Here's how the part is built. I have some questions about the finished solid (model axes, mm). A direction names the side the tool comes from. Round coordinates to 2 decimals unless told otherwise and drop trailing zeros. Write each loop counter-clockwise with the first axis right and the second up, starting at its lowest first coordinate (ties: lowest second). Pieces come first, ordered by that corner, then holes. Notation, with made-up numbers: M 69,18.5 L 109,18.5 A19 ccw 109,44.5 Z; hole C 79.5,49.5 d4. An arc over 180 degrees is marked long. Use one line per item in the form item = value. Start each with the question number.
Q1. I want a section at D-D on x = 25. List the corners of the cut face in (y, z) for me, and give its area (3 significant figures).
Q2. I'm going to push a flat-ended pin straight in: pin 1 Ø1 at (y, z) = (-6.5, -0.5) entering from -X. Where does the tip first touch, or does it pass through?
Q3. I want a section at B-B on y = 0. List the corners of the cut face in (x, z) for me.
Q4. We'd pull the mould along X, two halves only. Please class faces 1 (the face through (-30.745, -1.854, 0.018)), 2 (the face through (26.52, 10.27, 0.02)), 3 (the face through (-11.436, -0.3, 0.018)): +X half, -X half, draft (parallel to the pull), parting line (faces both ways), or undercut.
Q5. For faces 4 (the face through (-27.201, -1.222, 0.018)), 5 (the face through (26.34, -10.4, 0.02)), which set-ups out of +Z, -Z, +X, -X, +Y, -Y let a thin tool reach every point of the face, with its end or its side?
Q6. I need wall thicknesses on line 1 along Y through (x, z) = (19.05, -0.5); line 2 along X through (y, z) = (4, 0.9); line 3 along X through (y, z) = (0.5, 0.6). Which ranges of each line are inside material? Lowest first, please. Write a range as from..to.
Q7. I want a section at C-C on y = -6.25. List the corners of the cut face in (x, z) for me, and give its area (3 significant figures).
```python
from build123d import *

# Parameters (mm, degrees)
F1_DEPTH = 1.27
F2_R     = 7.62
F3_DEPTH = 25.4
F5_W     = 12.5357808316
F5_H     = 1.524
F6_DEPTH = 25.4
F7_R     = 2.53999


# Not quite as in the source:
# - a fillet or chamfer is up to 0.001 mm smaller than in the source, because OpenCascade refuses the exact size


with BuildPart() as f1:
    # F0 (on Top) → F1 (new body, symmetric)
    with BuildSketch(Plane.XY):
        with BuildLine():
            Line((19.05, 12.7), (-19.05, 12.7))
            ThreePointArc((-19.05, 12.7), (-31.75, 0), (-19.05, -12.7))
            Line((-19.05, -12.7), (19.05, -12.7))
            ThreePointArc((19.05, -12.7), (31.75, 0), (19.05, 12.7))
        make_face()
    extrude(amount=F1_DEPTH, both=True)

    # F2 (on face) → F3 (cut)
    with BuildSketch(Plane.XY.offset(1.27)):
        with Locations((-19.05, 0)):
            Circle(F2_R)
        with Locations((19.05, 0)):
            Circle(F2_R)
        with BuildLine():
            Line((8.89, 7.62), (-8.89, 7.62))
            ThreePointArc((-8.89, 7.62), (-6.35, 0), (-8.89, -7.62))
            Line((-8.89, -7.62), (8.89, -7.62))
            ThreePointArc((8.89, -7.62), (6.35, 0), (8.89, 7.62))
        make_face()
    extrude(amount=-F3_DEPTH, mode=Mode.SUBTRACT)

    # F5 (on face) → F6 (cut)
    with BuildSketch(Plane.XY.offset(1.27)):
        with Locations((-25.4821095842, 0)):
            Rectangle(F5_W, F5_H)
        with Locations((25.4821095842, 0)):
            Rectangle(F5_W, F5_H)
    extrude(amount=-F6_DEPTH, mode=Mode.SUBTRACT)

    # F7 (radius 2.54 in the source; OpenCascade refuses exactly that, so slightly less here)
    f7_edges = [f1.edges().sort_by_distance(p)[0] for p in [
        (26.631804, 0.762, 0),
        (26.631804, -0.762, 0),
        (-26.631804, 0.762, 0),
        (-26.631804, -0.762, 0),
        (-31.727119, -0.762, 0),
        (-31.727119, 0.762, 0),
        (31.727119, 0.762, 0),
        (31.727119, -0.762, 0),
    ]]
    fillet(f7_edges, radius=F7_R)


solid = f1.part
```
Reported:
q1.outline = M -11.22,-1.27 L -4.76,-1.27 L -4.76,1.27 L -11.22,1.27 Z; M 4.76,-1.27 L 11.22,-1.27 L 11.22,1.27 L 4.76,1.27 Z
q1.area = 32.8 mm^2
q2.pin_1 = -30.24
q3.outline = M -11.43,-1.27 L -6.35,-1.27 L -6.35,1.27 L -11.43,1.27 Z; M 6.35,-1.27 L 11.43,-1.27 L 11.43,1.27 L 6.35,1.27 Z
q4.face_1 = -X half
q4.face_2 = +X half
q4.face_3 = undercut
q5.face_4 = +Z, -Z
q5.face_5 = +Z, -Z, +X, -Y
q6.line_1 = -12.7..-7.62, 7.62..12.7
q6.line_2 = -31.1..-25.54, -12.56..-7, 7..12.56, 25.54..31.1
q6.line_3 = -11.45..-6.36, 6.36..11.45
q7.outline = M -30.11,-1.27 L -23.41,-1.27 L -23.41,1.27 L -30.11,1.27 Z; M -14.69,-1.27 L -7.99,-1.27 L -7.99,1.27 L -14.69,1.27 Z; M 7.99,-1.27 L 14.69,-1.27 L 14.69,1.27 L 7.99,1.27 Z; M 23.41,-1.27 L 30.11,-1.27 L 30.11,1.27 L 23.41,1.27 Z
q7.area = 68.0 mm^2
